Autodesk Inventor part; units mm, degrees
ref_plane "YZ Plane" through (0, 0, 0) normal (1, 0, 0) x (0, 1, 0)
ref_plane "XZ Plane" through (0, 0, 0) normal (0, 1, 0) x (-1, 0, 0)
ref_plane "XY Plane" through (0, 0, 0) normal (0, 0, 1) x (1, 0, 0)
sketch "Sketch1" plane through (0, 0, 0) normal (0, 0, 1) x (1, 0, 0)
  line L0 (0, 0) -> (20, 0)
  line L1 (20, 0) -> (20, 16)
  line L2 (20, 16) -> (15, 16)
  line L3 (15, 16) -> (15, 5)
  line L4 (15, 5) -> (0, 5)
  line L5 (0, 5) -> (0, 0)
  line L6 (20, 0) -> (15, 0)
  line L7 (15, 0) -> (15, -4)
  line L8 (15, -4) -> (20, -4)
  line L9 (20, -4) -> (20, 0)
  dimension "d0" = 5
  dimension "d1" = 20
  dimension "d2" = 5
  dimension "d3" = 16
  dimension "d4" = 20
extrude "Extrusion1" add sketch "Sketch1" along normal blind 320
mirror "Mirror1" about plane through (0, 0, 0) normal (1, 0, 0) of "Extrusion1"
ref_plane "Work Plane1" through (0, 0, 160) normal (0, 0, 1) x (1, 0, 0)
sketch "Sketch3" plane through (0, 0, 0) normal (0, 0, -1) x (-1, 0, 0)
  line L0 (20, -4) -> (20, 16)
  line L1 (-15, -4) -> (-20, -4)
  line L2 (20, 16) -> (-20, 16)
  line L3 (-20, 16) -> (-20, -4)
  line L4 (-20, -4) -> (20, -4)
  line L5 (20, -4) -> (20, 16)
  point P0 (0, 0)
extrude "Extrusion2" add sketch "Sketch3" along normal blind 10
ref_plane "Work Plane2" through (0, -4, 320) normal (-1, 0, 0) x (0, 0, 1)
sketch "Sketch4" plane through (-15, 16, 0) normal (0, 1, 0) x (1, 0, 0)
  line L0 (15, -386) -> (15, 76)
  point P0 (15, 0)
  point P1 (0, 4.6383)
  point P2 (30, 4.6383)
  dimension "d9" = 30
  dimension "d10" = 15
hole "Hole1" at (-15, 16, -4.6383) at (15, 16, -4.6383) direction (0, -1, 0) diameter 5 end through all
mirror "Mirror3" about plane through (0, 0, 160) normal (0, 0, 1) of "Extrusion2", "Hole1"
sketch "Sketch5" plane through (-20, 16, -10) normal (0, 1, 0) x (1, 0, 0)
  line L0 (35, -330) -> (5, -330)
  line L1 (0, -340) -> (40, -340)
  line L2 (30, -330) -> (10, -330)
  line L3 (10, -330) -> (10, -340)
  line L4 (10, -340) -> (30, -340)
  line L5 (30, -340) -> (30, -330)
  line L6 (20, -396) -> (20, 66)
  point P0 (20, -10)
  point P1 (20, -340)
  point P2 (20, -330)
  dimension "d18" = 20
  dimension "d31" = 10
extrude "Extrusion3" cut sketch "Sketch5" against normal blind 10
sketch "Sketch6" plane through (-20, 6, -10) normal (0, 1, 0) x (1, 0, 0)
  line L0 (30, -340) -> (10, -340)
  line L1 (30, -330) -> (30, -340)
  point P0 (20, -10)
  point P1 (24.8, -336)
  point P2 (15.3, -336)
  dimension "d21" = 4
  dimension "d22" = 9.5
  dimension "d30" = 5.2
hole "Hole2" at (4.8, 6, 326) at (-4.7, 6, 326) direction (0, -1, 0) diameter 2.3 end through all
mirror "Mirror4" about plane through (0, 0, 160) normal (0, 0, 1) of "Hole2", "Extrusion3"
sketch "Sketch7" plane through (-20, -4, 330) normal (0, 0, 1) x (1, 0, 0)
  line L0 (10, 20) -> (10, 10)
  line L1 (10, 20) -> (0, 20)
  line L2 (0, 20) -> (0, 0)
  line L3 (0, 0) -> (10, 0)
  line L4 (10, 0) -> (10, 20)
  line L5 (40, 0) -> (0, 0)
  line L6 (0, 0) -> (0, 20)
  point P0 (20, 4)
  point P1 (10, 10)
extrude "Extrusion4" add sketch "Sketch7" along normal blind 30
mirror "Mirror6" about plane through (0, 0, 160) normal (0, 0, 1) of "Extrusion4"
mirror "Mirror7" about plane through (0, -4, 320) normal (-1, 0, 0) of "Extrusion4", "Mirror6"
sketch "Sketch10" plane through (-10, -4, 330) normal (1, 0, 0) x (0, 0, -1)
  line L0 (-10, 10) -> (-25, 10) construction
  line L1 (-10, 12.5) -> (-25, 12.5)
  line L2 (-25, 7.5) -> (-10, 7.5)
  arc A0 (-10, 7.5) -> (-10, 12.5) centre (-10, 10) ccw
  arc A1 (-25, 12.5) -> (-25, 7.5) centre (-25, 10) ccw
  line L3 (-30, 0) -> (-30, 20)
  line L4 (0, 0) -> (-30, 0)
  point P0 (330, 4)
  point P1 (-17.5, 10)
  dimension "d45" = 2.5
  dimension "d46" = 15
  dimension "d47" = 5
  dimension "d48" = 10
extrude "Extrusion6" cut sketch "Sketch10" against normal through all
mirror "Mirror5" about plane through (0, -4, 320) normal (-1, 0, 0) of "Extrusion4", "Extrusion6"
sketch "Sketch9" plane through (-20, -4, -10) normal (0, -1, 0) x (1, 0, 0)
  line L0 (10, 340) -> (10, 370)
  line L1 (30, 330) -> (30, 340)
  line L2 (10, 340) -> (30, 340)
  line L3 (30, 340) -> (30, 330)
  line L4 (30, 330) -> (10, 330)
  line L5 (10, 330) -> (10, 340)
  point P0 (20, 10)
extrude "Extrusion5" cut sketch "Sketch9" against normal up to surface (4 mm away)
sketch "Sketch11" plane through (-20, -4, 360) normal (-1, 0, 0) x (0, 0, 1)
  line L0 (-400, 20) -> (-400, 0)
  line L1 (0, 20) -> (-400, 20)
  point P0 (-360, 4)
  point P1 (-395, 10)
  point P2 (-400, 10)
  dimension "d51" = 5
  dimension "d52" = 10
hole "Hole4" at (-20, 6, -35) direction (1, 0, 0) diameter 5 end through all
properties part number "Sledge_rail" material "PC/ABS Plastic"
CAD build for the part. Positions are in the model's coordinates, mm. A direction names the side the tool comes from. Give positions to 0.01 mm unless a question says otherwise; leave off trailing zeros. Order: outer loops, then holes, each group sorted by start corner. A loop starts at its lowest first (then second) coordinate and runs counter-clockwise, first axis right, second up. Notation, with made-up numbers: M 60.25,25.5 L 100.25,25.5 A8 ccw 100.25,36.5 Z; hole C 1.25,-0.5 d11. An arc over 180 degrees is marked long. Put each result on its own line as item: value. Start each with the question number.
(1) Saw through at A-A, the plane z = 7.5. Write the cut outline in (x, y), then the cut area to 3 significant figures.
(2) Which spindle directions (+Z, -Z, +X, -X, +Y, -Y) get a long thin tool onto all of the face, cutting with end or side? Do faces 1 (the flat face through (0, 6, 325)), 2 (the flat face through (-16, 16, 163)), 3 (the flat face through (15, 3.5, 347)), 4 (the flat face through (-15, 6, -40)), 5 (the flat face through (-15, 10, 158)). Say none if no direction does.
(3) Mould opens along Z. For faces 6 (the flat face through (-15, 6, 360)), 7 (the flat face through (15, 6, -40)), 8 (the flat face through (-10, 6, 335)), 9 (the flat face through (15, 8.5, 348)) say: +Z half, -Z half, draft (parallel to the pull), parting line (faces both ways), or undercut.
(4) Flat gauge pins, fed straight in: pin 1 Ø12 at (x, z) = (2.5, 302) entering from -Y; pin 2 Ø5 at (x, z) = (3.5, -5.5) entering from +Y; pin 3 Ø1 at (x, z) = (-6.5, 58) entering from +Y. Where does each tip first touch, or does it go through?
(5) Drill centre lines: line 1 along X through (y, z) = (-0.25, 337.5); line 2 along Y through (x, z) = (-15, -35); line 3 along X through (y, z) = (6.25, 106.5). Where is each one in solid material? Low to high.
Check result:
1. outline: M -20,-4 L -15,-4 L -15,0 L 15,0 L 15,-4 L 20,-4 L 20,16 L 15,16 L 15,5 L -15,5 L -15,16 L -20,16 Z
1. area: 350 mm2
2. face 1: +Z, -Z, +Y
2. face 2: +Z, -Z, +X, -X, +Y
2. face 3: +X, -X
2. face 4: -Z, +X, -X, +Y, -Y
2. face 5: +Y
3. face 6: +Z half
3. face 7: -Z half
3. face 8: draft
3. face 9: undercut
4. pin 1: stops at y = 0
4. pin 2: stops at y = 6
4. pin 3: stops at y = 5
5. line 1: x = -20 to -10, 10 to 20
5. line 2: y = -4 to 3.5, 8.5 to 16
5. line 3: x = -20 to -15, 15 to 20
